from build123d import *

# Parameters (mm, degrees)
BOSS_EXTRUDE1_DEPTH = 12.605
CUT_EXTRUDE1_DEPTH  = 32.2
SKETCH3_R           = 3.935
SKETCH3_R_2         = 1
CUT_EXTRUDE2_DEPTH  = 32.2
BOSS_EXTRUDE2_DEPTH = 21.39
SKETCH6_R           = 0.5
SKETCH6_W           = 16.3
SKETCH6_H           = 38.2
CUT_EXTRUDE4_DEPTH  = 45
CUT_EXTRUDE5_DEPTH  = 68
CHAMFER3_SIZE       = 2


with BuildPart() as part:
    # Sketch1 → Boss-Extrude1 (new, symmetric)
    with BuildSketch(Plane(origin=(0, 0, 0), x_dir=(1, 0, 0), z_dir=(0, 1, 0))):
        Polygon((0, 0), (-21.71, 0), (-21.71, -63.54), (-20, -63.54), (-20, -1.71), (0, -1.71), align=None)
    boss_extrude1 = extrude(amount=BOSS_EXTRUDE1_DEPTH, both=True)

    # Sketch2 → Cut-Extrude1 (cut)
    with BuildSketch(Plane.ZY.offset(21.71)):
        Polygon((57.565, 12.605), (63.54, 6.63), (63.54, 12.605), align=None)
        Polygon((63.54, -6.63), (57.565, -12.605), (63.54, -12.605), align=None)
    cut_extrude1 = extrude(amount=-CUT_EXTRUDE1_DEPTH, mode=Mode.SUBTRACT)

    # Sketch3 → Cut-Extrude2 (cut)
    with BuildSketch(Plane.ZY.offset(21.71)):
        with Locations((50.77, 0)):
            Circle(SKETCH3_R)
        with Locations((45.77, 5)):
            Circle(SKETCH3_R_2)
        with Locations((55.77, 5)):
            Circle(SKETCH3_R_2)
        with Locations((55.77, -5)):
            Circle(SKETCH3_R_2)
        with Locations((45.77, -5)):
            Circle(SKETCH3_R_2)
        with Locations((43.698932188, 0)):
            Circle(SKETCH3_R_2)
        with Locations((50.77, -7.071067812)):
            Circle(SKETCH3_R_2)
        with Locations((57.841067812, 0)):
            Circle(SKETCH3_R_2)
        with Locations((50.77, 7.071067812)):
            Circle(SKETCH3_R_2)
    cut_extrude2 = extrude(amount=-CUT_EXTRUDE2_DEPTH, mode=Mode.SUBTRACT)

    # Mirror1: Boss-Extrude1, Cut-Extrude1, Cut-Extrude2 across plane
    add(boss_extrude1.mirror(Plane(origin=(0, 12.605, 1.71), x_dir=(0, 0, 1), z_dir=(-1, 0, 0))))
    add(cut_extrude1.mirror(Plane(origin=(0, 12.605, 1.71), x_dir=(0, 0, 1), z_dir=(-1, 0, 0))), mode=Mode.SUBTRACT)
    add(cut_extrude2.mirror(Plane(origin=(0, 12.605, 1.71), x_dir=(0, 0, 1), z_dir=(-1, 0, 0))), mode=Mode.SUBTRACT)

    # Sketch5 → Boss-Extrude2 (add)
    with BuildSketch(Plane.XZ.offset(12.605)):
        Polygon((-21.71, 28.8), (-20, 28.8), (-20, 1.71), (20, 1.71), (20, 28.8), (21.71, 28.8), (21.71, 0), (-21.71, 0), align=None)
    extrude(amount=BOSS_EXTRUDE2_DEPTH)

    # Sketch6 → Cut-Extrude4 (cut)
    with BuildSketch(Plane(origin=(0, 0, 0), x_dir=(-1, 0, 0), z_dir=(0, 0, -1))):
        with Locations((-9.25, 9.305)):
            Circle(SKETCH6_R)
        with Locations((9.25, 9.305)):
            Circle(SKETCH6_R)
        with Locations((9.25, -30.695)):
            Circle(SKETCH6_R)
        with Locations((-9.25, -30.695)):
            Circle(SKETCH6_R)
        Polygon((-21.71, -26.845), (-21.71, -33.995), (-13.96, -33.995), (-13.96, -26.845), (-21.71, -23.295), align=None)
        Polygon((21.71, -23.295), (13.96, -26.845), (13.96, -33.995), (21.71, -33.995), (21.71, -26.845), align=None)
        with Locations((0, -10.695)):
            Rectangle(SKETCH6_W, SKETCH6_H)
    extrude(amount=-CUT_EXTRUDE4_DEPTH, mode=Mode.SUBTRACT)

    # Sketch7 → Cut-Extrude5 (cut)
    with BuildSketch(Plane(origin=(21.71, 0, 0), x_dir=(0, 0, -1), z_dir=(1, 0, 0))):
        Polygon((-28.8, -12.605), (-1.71, -23.295), (-1.71, -35.593839202), (-28.8, -35.593839202), align=None)
    extrude(amount=-CUT_EXTRUDE5_DEPTH, mode=Mode.SUBTRACT)

    # Chamfer3
    chamfer3_edges = [part.edges().sort_by_distance(p)[0] for p in [
        (-8.15, 8.405, 0.855),
        (-8.15, -29.795, 0.855),
        (8.15, -29.795, 0.855),
        (8.15, 8.405, 0.855),
    ]]
    chamfer(chamfer3_edges, length=CHAMFER3_SIZE)


solid = part.part
Source: CAD feature listing. Evaluate the final solid. Frame: model axes, mm. A direction names the side the tool comes from. Round coordinates to 2 decimals unless told otherwise and drop trailing zeros. Loops run counter-clockwise (first coordinate to the right, second up) from the corner with the lowest first, then second, coordinate; pieces in that order, holes last. Notation, with made-up numbers: (13, -3) - (29, -3) arc R8 cw to (29, 7) - close; hole circle Ø4 at (6, 21.25). An arc over 180 degrees is marked (long way). Write item = value, one per line. Start each with the question number.
Item 1: Material intervals for line 1 (Y direction, x = 20.4, z = 45.77) (3 decimals); line 2 (Z direction, x = 21, y = 0) (3 decimals); line 3 (X direction, y = -1, z = 44), sorted ascending.
Item 2: Section query B-B on z = 50.77. Count the separate pieces of the cut face and the enclosed holes in it, plus the area to 3 significant figures.
Item 3: Section query C-C on y = 5. Output: boundary loops of the cut face in (x, z), plus the area to 3 significant figures.
Item 4: Section query A-A on x = -4. Output: boundary loops of the cut face in (y, z) (3 decimals).
Item 5: Section query D-D on z = 28. Output: boundary loops of the cut face in (x, y) (3 decimals).
Item 6: First-contact query: pin 1 Ø1.4 at (x, z) = (20.5, 41.5) entering from -Y (3 decimals); pin 2 Ø21.5 at (x, y) = (-6.5, -5.5) entering from +Z. Flat tips, straight axial feed; report the tip coordinate or a pass-through.
Item 7: Reachability of faces 4 (the face through (0, 8.405, 1)), 5 (the face through (-21, -12.605, 43)), 6 (the face through (13.96, -30, 1)) from +Z, -Z, +X, -X, +Y, -Y: full face, straight path, thin tool, end or side. Return the list, or none.
Item 8: Mould query, pull axis X, two halves, no side actions, for faces 1 (the face through (-20, -1, 33)), 2 (the face through (-17.889, -25.045, 0.843)), 3 (the face through (-20.867, 5.3, 56.724)). Classes: released by +X, released by -X, zero draft, split by the parting line, or undercut.
Results list:
q1.line_1 = -12.605 to -6, -4 to 4, 6 to 12.605
q1.line_2 = 0 to 42.699, 44.699 to 46.835, 54.705 to 56.841, 58.841 to 63.54
q1.line_3 = -21.71 to -20, 20 to 21.71
q2.separate_pieces = 8
q2.enclosed_holes = 0
q2.area = 45.6 mm²
q3.outline = (-21.71, 0) - (-8.15, 0) - (-8.15, 1.71) - (-20, 1.71) - (-20, 44.77) - (-21.71, 44.77) - close; (-21.71, 46.77) - (-20, 46.77) - (-20, 54.77) - (-21.71, 54.77) - close; (-21.71, 56.77) - (-20, 56.77) - (-20, 63.54) - (-21.71, 63.54) - close; (8.15, 0) - (21.71, 0) - (21.71, 44.77) - (20, 44.77) - (20, 1.71) - (8.15, 1.71) - close; (20, 46.77) - (21.71, 46.77) - (21.71, 54.77) - (20, 54.77) - close; (20, 56.77) - (21.71, 56.77) - (21.71, 63.54) - (20, 63.54) - close
q3.area = 244 mm²
q4.outline = (-33.995, 0) - (-29.795, 0) - (-29.795, 1.71) - (-33.995, 1.71) - close; (8.405, 0) - (12.605, 0) - (12.605, 1.71) - (8.405, 1.71) - close
q5.outline = (-21.71, -12.921) - (-20, -12.921) - (-20, 12.605) - (-21.71, 12.605) - close; (20, -12.921) - (21.71, -12.921) - (21.71, 12.605) - (20, 12.605) - close
q6.pin_1 = -12.605
q6.pin_2 = 1.71
q7.face_4 = +Z, -Z
q7.face_5 = +Z, +X, -X, -Y
q7.face_6 = +Z, -Z, +X, -Y
q8.face_1 = undercut
q8.face_2 = released by -X
q8.face_3 = zero draft
